```python
from build123d import *

# Parameters (mm, degrees)
F0_R          = 12.5
F1_DEPTH      = 30
F2_R          = 5
F3_DEPTH      = 20
F4_R          = 3.15
F5_DEPTH      = 10
F6_W          = 10
F6_H          = 22
F7_DEPTH      = 0.5
F7_DEPTH_BACK = 0.5
F8_R          = 3
F9_DEPTH      = 12.501


with BuildPart() as f1:
    # F0 (on Front) → F1 (new body)
    with BuildSketch(Plane.XZ):
        Circle(F0_R)
    extrude(amount=-F1_DEPTH)

    # F2 (on face) → F3 (cut)
    with BuildSketch(Plane.XZ):
        Circle(F2_R)
    extrude(amount=-F3_DEPTH, mode=Mode.SUBTRACT)

    # F4 (on face) → F5 (cut, through all)
    with BuildSketch(Plane(origin=(0, 30, 0), x_dir=(-1, 0, 0), z_dir=(0, 1, 0))):
        Circle(F4_R)
    extrude(amount=-F5_DEPTH, mode=Mode.SUBTRACT)

    # F6 (on Right) → F7 (cut, two sides)
    with BuildSketch(Plane.YZ) as f7_sk:
        with Locations((5, 1.5)):
            Rectangle(F6_W, F6_H)
        with Locations((25, 1.5)):
            Rectangle(F6_W, F6_H)
    extrude(amount=-F7_DEPTH, mode=Mode.SUBTRACT)
    extrude(f7_sk.sketch, amount=F7_DEPTH_BACK, mode=Mode.SUBTRACT)

    # F8 (on Right) → F9 (cut, through all)
    with BuildSketch(Plane.YZ):
        with Locations((5, 8.5)):
            Circle(F8_R)
        with Locations((25, 8.5)):
            Circle(F8_R)
    extrude(amount=-F9_DEPTH, mode=Mode.SUBTRACT)


solid = f1.part
```
Could you check a few things on this model? Use its own coordinates, in mm. A direction names the side the tool comes from. Give positions to 0.01 mm unless a question says otherwise; leave off trailing zeros. Loops run counter-clockwise (first coordinate to the right, second up) from the corner with the lowest first, then second, coordinate; pieces in that order, holes last. Notation, with made-up numbers: (4.5, -24.5) - (9.5, -24.5) arc R30 cw to (9.5, 14.5) - close; hole circle Ø8 at (-8, 43.25). An arc over 180 degrees is marked (long way). Use one line per item in the form item = value.
1. I need wall thicknesses on probe 1 along Y at (x, z) = (-3.5, 8.5); probe 2 along Z at (x, y) = (0, 13). Which ranges of each line are inside material? Lowest first, please.
Response values:
probe_1 = 0 to 2, 8 to 22, 28 to 30
probe_2 = -12.5 to -5, 5 to 12.5
2. I'm going to push flat-ended pins straight in: pin 1 Ø0.5 at (x, z) = (0, 9) entering from +Y; pin 2 Ø2.5 at (y, z) = (2.5, -8) entering from +X; pin 3 Ø8.5 at (y, z) = (2.5, 9.5) entering from -X. Where does each tip first touch, or does it pass through?
Response values:
pin_1 = 20
pin_2 = 10.52
pin_3 = -11.34
3. I want a section at B-B (x = 0). Please give me the cut outline in (y, z).
Response values:
outline = (0, -12.5) - (30, -12.5) - (30, -9.5) - (20, -9.5) - (20, -5) - (10, -5) - (10, -9.5) - (0, -9.5) - close; (10, 5) - (20, 5) - (20, 12.5) - (10, 12.5) - close
4. I want a section at D-D (z = 8.5). Please give me the cut outline in (x, y).
Response values:
outline = (-9.17, 0) - (-0.5, 0) - (-0.5, 2) - (-9.17, 2) - close; (-9.17, 8) - (-0.5, 8) - (-0.5, 10) - (0.5, 10) - (0.5, 0) - (9.17, 0) - (9.17, 30) - (0.5, 30) - (0.5, 20) - (-0.5, 20) - (-0.5, 22) - (-9.17, 22) - close; (-9.17, 28) - (-0.5, 28) - (-0.5, 30) - (-9.17, 30) - close
5. On a 3-axis mill with a long thin cutter (end or side, diameter ignored), from which of +Z, -Z, +X, -X, +Y, -Y can I reach the whole of each face in a straight line? I mean faces 1 (the face through (-4.6, 24.35, 5.57)), 2 (the face through (3.15, 25.07, 0.06)), 3 (the face through (0.5, 5, -7)). Say none if no direction works.
Response values:
face_1 = -X
face_2 = +Y, -Y
face_3 = +Z, -Y
6. Thinking about a two-plate mould opening in Y: for faces 4 (the face through (0, 10, -7)), 5 (the face through (0.5, 25, -6)), 6 (the face through (-4.6, 4.35, 5.57)), which applies, released by +Y, released by -Y, zero draft, split by the parting line, or undercut?
Response values:
face_4 = released by -Y
face_5 = zero draft
face_6 = undercut
7. I want a section at C-C (y = 21). Please give me the cut outline in (x, z), and give its area (3 significant figures).
Response values:
outline = (-0.5, -9.5) - (-0.5, -3.11) arc R3.15 cw to (-0.5, 3.11) - (-0.5, 12.49) arc R12.5 ccw (long way) to (0.5, 12.49) - (0.5, 3.11) arc R3.15 cw to (0.5, -3.11) - (0.5, -9.5) - close
area = 444 mm²
8. I want a section at A-A (z = 0). Please give me the cut outline in (x, y), and give its area (3 significant figures).
Response values:
outline = (-12.5, 0) - (-5, 0) - (-5, 20) - (-3.15, 20) - (-3.15, 30) - (-12.5, 30) - close; (3.15, 20) - (5, 20) - (5, 0) - (12.5, 0) - (12.5, 30) - (3.15, 30) - close
area = 487 mm²
